```python
from build123d import *

# Parameters (mm, degrees)
F0_W     = 10
F0_H     = 180
F1_DEPTH = 12.5
F3_DEPTH = 180.001
F5_ANGLE = 90
F6_R     = 2.5
F7_DEPTH = 10.001


with BuildPart() as f1:
    # F0 (on Front) → F1 (new body, symmetric)
    with BuildSketch(Plane.XZ):
        Rectangle(F0_W, F0_H)
    extrude(amount=F1_DEPTH, both=True)

    # F2 (on face) → F3 (cut, through all)
    with BuildSketch(Plane.XY.offset(90)):
        with BuildLine():
            Line((-5, 12.5), (-5, -12.5))
            ThreePointArc((-5, -12.5), (0, 0), (-5, 12.5))
        make_face()
    extrude(amount=-F3_DEPTH, mode=Mode.SUBTRACT)


with BuildPart() as f1_1:
    # F5: moved
    add(f1.part.rotate(Axis((0, 0, 28.159656), (0, 0, -1)), F5_ANGLE))

    # F6 (on face) → F7 (cut, through all)
    with BuildSketch(Plane.XZ.offset(5)):
        with Locations((0, 10)):
            Circle(F6_R)
        with Locations((0, -60)):
            Circle(F6_R)
    extrude(amount=-F7_DEPTH, mode=Mode.SUBTRACT)


solid = f1_1.part
```
Part model, mm, in its own coordinate system. Round coordinates to 2 decimals unless told otherwise and drop trailing zeros. Loops run counter-clockwise (first coordinate to the right, second up) from the corner with the lowest first, then second, coordinate; pieces in that order, holes last.
Item 1: Drill centre lines: line 1 (Z direction, x = 0, y = -1.2); line 2 (X direction, y = -1.2, z = -60); line 3 (Y direction, x = 2.5, z = -33). Where is each one in solid material? Low to high.
Item 2: Mould opens along X. For faces 1 (the face through (-0.54, -2.45, 7.56)), 2 (the face through (12.5, 0, 1)), 3 (the face through (0, -1, 90)), 4 (the face through (0, 0, 1)) say: +X half, -X half, draft (parallel to the pull), parting line (faces both ways), or undercut.
Item 3: Cut at D-D, the plane x = 6.75. Give the cut face in (y, z), then the cut area to 3 significant figures.
Item 4: Cut at A-A, the plane z = 10. Give the cut face in (x, y) (3 decimals).
Item 5: Cut at B-B, the plane x = 0. Give the cut face in (y, z), then the cut area to 3 significant figures.
Item 6: Drop flat-ended pins along their axis: P1, Ø12, axis at x = -3, z = -13, coming from the +Y side; P2, Ø5, axis at x = -1.5, z = -27, coming from the +Y side; P3, Ø2, axis at x = 5, z = -46.5, coming from the +Y side; P4, Ø2, axis at x = -3.5, y = 1, coming from the +Z side. Give the stop position or say it passes through.
Item 7: Cut at C-C, the plane z = -64.5. Give the cut face in (x, y) (3 decimals).
A:
1. line 1: z = -90 to -62.5, -57.5 to 7.5, 12.5 to 90
1. line 2: x = -12.5 to -2.5, 2.5 to 12.5
1. line 3: y = -5 to 0.17
2. face 1: undercut
2. face 2: +X half
2. face 3: draft
2. face 4: undercut
3. outline: (-5, -90) - (1.3, -90) - (1.3, 90) - (-5, 90) - close
3. area: 1,130 mm2
4. outline: (-12.5, -5) - (-2.5, -5) - (-2.5, 0.173) arc R18.125 cw to (-12.5, 5) - close; (2.5, -5) - (12.5, -5) - (12.5, 5) arc R18.125 cw to (2.5, 0.173) - close
5. outline: (-5, -90) - (0, -90) - (0, -62.5) - (-5, -62.5) - close; (-5, -57.5) - (0, -57.5) - (0, 7.5) - (-5, 7.5) - close; (-5, 12.5) - (0, 12.5) - (0, 90) - (-5, 90) - close
5. area: 850 mm2
6. P1: stops at y = 2.39
6. P2: stops at y = 0.45
6. P3: stops at y = 1.02
6. P4: stops at z = 90
7. outline: (-12.5, -5) - (12.5, -5) - (12.5, 5) arc R18.125 cw to (-12.5, 5) - close
